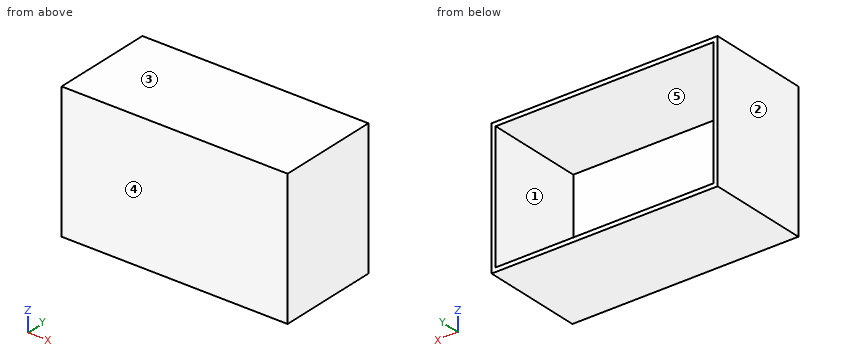
from build123d import *

# Parameters (mm, degrees)
SKETCH1_W           = 698.5
SKETCH1_H           = 419.1
BOSS_EXTRUDE1_DEPTH = 12.7
SKETCH1_3_W         = 698.5
SKETCH1_3_H         = 419.1
SKETCH1_3_W_2       = 673.1
SKETCH1_3_H_2       = 393.7
BOSS_EXTRUDE2_DEPTH = 304.8


with BuildPart() as part:
    # Sketch1 → Boss-Extrude1 (new body)
    with BuildSketch(Plane(origin=(0, 0, 0), x_dir=(1, 0, 0), z_dir=(0, 1, 0))):
        Rectangle(SKETCH1_W, SKETCH1_H)
    extrude(amount=-BOSS_EXTRUDE1_DEPTH)

    # Sketch1<3> → Boss-Extrude2 (add)
    with BuildSketch(Plane(origin=(0, 0, 0), x_dir=(1, 0, 0), z_dir=(0, 1, 0))):
        Rectangle(SKETCH1_3_W, SKETCH1_3_H)
        Rectangle(SKETCH1_3_W_2, SKETCH1_3_H_2, mode=Mode.SUBTRACT)
    extrude(amount=BOSS_EXTRUDE2_DEPTH)


solid = part.part
For this review, take the finished solid that the model builds, in its own axes (mm). Face numbers are marked on the shaded views. A direction names the side the tool comes from. Coordinates: 2 decimals unless noted, no trailing zeros. Order: outer loops, then holes, each group sorted by start corner. A loop starts at its lowest first (then second) coordinate and runs counter-clockwise, first axis right, second up. Notation, with made-up numbers: (68.5, 31) -> (88.5, 31) arc R16 cw to (88.5, 41) -> close; hole circle Ø3 at (0, -0.75). An arc over 180 degrees is marked (long way). Return JSON: item names as keys, results as strings.
1. Machinability: for the marked faces 4 and 5, which of the approach directions +Z, -Z, +X, -X, +Y, -Y give a long, thin tool a straight path to every point of the face, cutting with its end or side? Answer none if there is none.
Answer block:
{"face 4": "+Z, -Z, +X, -X, -Y", "face 5": "+Y"}
2. For line 1 (X direction, y = 27, z = 102); line 2 (Z direction, x = -78, y = 39); line 3 (Y direction, x = 104, z = -174), list the stretches that pass through material, from the lowest coordinate up. Write a range as from..to.
Answer block:
{"line 1": "-349.25..-336.55, 336.55..349.25", "line 2": "-209.55..-196.85, 196.85..209.55", "line 3": "-12.7..0"}
3. For pin 1 Ø3 at (x, z) = (-203, 63) entering from +Y, flat-tipped, find the tip position at first contact; note if it passes through.
Answer block:
{"pin 1": "y = 0"}
4. We need section A-A on z = 110.5. Write out the cut boundary in (x, y), and give its area (3 significant figures).
Answer block:
{"outline": "(-349.25, -12.7) -> (349.25, -12.7) -> (349.25, 304.8) -> (336.55, 304.8) -> (336.55, 0) -> (-336.55, 0) -> (-336.55, 304.8) -> (-349.25, 304.8) -> close", "area": "16,600 mm²"}
5. The part is to be moulded in two halves that separate along X. For the marked faces 1, 2 and 3, say which applies: +X half, -X half, draft (parallel to the pull), parting line (faces both ways), or undercut.
Answer block:
{"face 1": "undercut", "face 2": "-X half", "face 3": "draft"}
6. We need section B-B on y = 264. Write out the cut boundary in (x, z), and give its area (3 significant figures).
Answer block:
{"outline": "(-349.25, -209.55) -> (349.25, -209.55) -> (349.25, 209.55) -> (-349.25, 209.55) -> close; hole (-336.55, -196.85) -> (336.55, -196.85) -> (336.55, 196.85) -> (-336.55, 196.85) -> close", "area": "27,700 mm²"}
7. We need section C-C on x = 101. Write out the cut boundary in (y, z).
Answer block:
{"outline": "(-12.7, -209.55) -> (304.8, -209.55) -> (304.8, -196.85) -> (0, -196.85) -> (0, 196.85) -> (304.8, 196.85) -> (304.8, 209.55) -> (-12.7, 209.55) -> close"}
